CAD build for the part. Positions are in the model's coordinates, mm. A direction names the side the tool comes from. Coordinates: 2 decimals unless noted, no trailing zeros. Write each loop counter-clockwise with the first axis right and the second up, starting at its lowest first coordinate (ties: lowest second). Pieces come first, ordered by that corner, then holes. Notation, with made-up numbers: (-34, -1.5) - (2, -1.5) arc R14 ccw to (2, 16.5) - close; hole circle Ø1 at (-18, 0). An arc over 180 degrees is marked (long way). Answer in a Markdown table with one row per item. Add a question column.
Q1. Two-plate mould, pull along Z, no slides. Class faces 6 (the cylindrical face through (26.36, 3.9, -5.13)), 7 (the cylindrical face through (-12.15, 49.02, -13.91)), 8 (the cylindrical face through (17.483, 49.021, -0.26)): +Z half, -Z half, draft (parallel to the pull), parting line (faces both ways), or undercut.
Q2. Pin check, flat tips, straight feed: pin 1 (5.5 mm diameter, centred on y = 29.5, z = -3.5, fed in from +X); pin 2 (1.5 mm diameter, centred on y = 7.5, z = -11.5, fed in from -X); pin 3 (5.5 mm diameter, centred on x = -34.5, z = -9.5, fed in from +Y). Stop position of each tip, or through.
Q3. Drill centre lines: line 1 along X through (y, z) = (48.9, 0); line 2 along X through (y, z) = (44.5, -6.5); line 3 along X through (y, z) = (1, -5). Where is each one in solid material? Low to high. Write a range as from..to.
Q4. 3-axis set-ups, long thin cutter, end or side, ignore diameter. For faces 1 (the cylindrical face through (38, 2, -5)), 2 (the flat face through (36, 3, -5)), 3 (the flat face through (22.5, 25, -5)), 4 (the cylindrical face through (12.11, 49.02, -13.88)), 5 (the flat face through (-36, 3, -5)): which of +Z, -Z, +X, -X, +Y, -Y reach the whole face in a straight line?
Q5. Band-saw the part on B-B (x = 40). List the corners of the cut face in (y, z).
Q6. Band-saw the part on C-C (z = -0.5). List the corners of the cut face in (x, y), and give its area (3 significant figures).
Q7. Band-saw the part on A-A (y = 33.5). List the corners of the cut face in (x, z).
Q8. Band-saw the part on D-D (z = -9.25). List the corners of the cut face in (x, y), and give its area (3 significant figures).
```python
from build123d import *

# Parameters (mm, degrees)
EXTRUDE_THIN1_DEPTH = 4.5
SKETCH2_R           = 2
CUT_EXTRUDE1_DEPTH  = 70.474815581
BOSS_EXTRUDE1_DEPTH = 10
SKETCH4_R           = 11.5
CUT_EXTRUDE2_DEPTH  = 71.829019476
FILLET1_R           = 3
FILLET2_R           = 3
SKETCH5_R           = 2
CUT_EXTRUDE3_DEPTH  = 69.722267134


with BuildPart() as part:
    # Sketch1 → Extrude-Thin1 (new, symmetric)
    with BuildSketch(Plane.XY):
        Polygon((-47.5, 0), (-22.5, 0), (-22.5, 47.5), (0, 47.5), (0, 50.5), (-25.5, 50.5), (-25.5, 3), (-47.5, 3), align=None)
    extrude_thin1 = extrude(amount=EXTRUDE_THIN1_DEPTH, both=True)

    # Mirror1: Extrude-Thin1 across plane
    add(extrude_thin1.mirror(Plane(origin=(0, 50.5, 4.5), x_dir=(0, 0, 1), z_dir=(1, 0, 0))))

    # Sketch2 → Cut-Extrude1 (cut, through all)
    with BuildSketch(Plane(origin=(0, 50.5, 0), x_dir=(1, 0, 0), z_dir=(0, 1, 0))):
        with Locations(Location((-15.5, 0, 0), (0, 0, 270))):
            Circle(SKETCH2_R)
        with Locations(Location((15.5, 0, 0), (0, 0, 270))):
            Circle(SKETCH2_R)
    extrude(amount=-CUT_EXTRUDE1_DEPTH, mode=Mode.SUBTRACT)

    # Sketch3 → Boss-Extrude1 (add)
    with BuildSketch(Plane(origin=(0, 0, -4.5), x_dir=(-1, 0, 0), z_dir=(0, 0, -1))):
        Polygon((-22.5, 47.5), (22.5, 47.5), (22.5, 0), (47.5, 0), (47.5, 3), (25.5, 3), (25.5, 50.5), (-25.5, 50.5), (-25.5, 3), (-47.5, 3), (-47.5, 0), (-22.5, 0), align=None)
    extrude(amount=BOSS_EXTRUDE1_DEPTH)

    # Sketch4 → Cut-Extrude2 (cut, through all)
    with BuildSketch(Plane(origin=(0, 50.5, 0), x_dir=(1, 0, 0), z_dir=(0, 1, 0))):
        with Locations((0, 15.5)):
            Circle(SKETCH4_R)
    extrude(amount=-CUT_EXTRUDE2_DEPTH, mode=Mode.SUBTRACT)

    # Fillet1
    fillet1_edges = [part.edges().sort_by_distance(p)[0] for p in [
        (-11.456439237, 49, -14.5),
        (11.456439237, 49, -14.5),
    ]]
    fillet(fillet1_edges, radius=FILLET1_R)

    # Fillet2
    fillet2_edges = [part.edges().sort_by_distance(p)[0] for p in [
        (-22.5, 0, -5),
        (-25.5, 3, -5),
        (22.5, 0, -5),
        (25.5, 3, -5),
    ]]
    fillet(fillet2_edges, radius=FILLET2_R)

    # Sketch5 → Cut-Extrude3 (cut, through all)
    with BuildSketch(Plane(origin=(0, 3, 0), x_dir=(1, 0, 0), z_dir=(0, 1, 0))):
        with Locations(Location((-40, 5, 0), (0, 0, 270))):
            Circle(SKETCH5_R)
        with Locations(Location((40, 5, 0), (0, 0, 270))):
            Circle(SKETCH5_R)
    extrude(amount=-CUT_EXTRUDE3_DEPTH, mode=Mode.SUBTRACT)


solid = part.part
```
Checked values:
| question | item | result |
|---|---|---|
| 1 | face 6 | draft |
| 1 | face 7 | -Z half |
| 1 | face 8 | undercut |
| 2 | pin 1 | stops at x = 25.5 |
| 2 | pin 2 | stops at x = -25.5 |
| 2 | pin 3 | stops at y = 3 |
| 3 | line 1 | x = -25.5..-17.5, -13.5..13.5, 17.5..25.5 |
| 3 | line 2 | x = -25.5..-22.5, 22.5..25.5 |
| 3 | line 3 | x = -47.5..-42, -38..-23.26, 23.26..38, 42..47.5 |
| 4 | face 1 | +Y, -Y |
| 4 | face 2 | +Z, -Z, +X, +Y |
| 4 | face 3 | +Z, -Z, -Y |
| 4 | face 4 | -Z, +Y, -Y |
| 4 | face 5 | +Z, -Z, -X, +Y |
| 5 | outline | (0, -14.5) - (3, -14.5) - (3, -7) - (0, -7) - close; (0, -3) - (3, -3) - (3, 4.5) - (0, 4.5) - close |
| 6 | outline | (-47.5, 0) - (-25.5, 0) arc R3 ccw to (-22.5, 3) - (-22.5, 47.5) - (-17.44, 47.5) - (-17.44, 50.5) - (-25.5, 50.5) - (-25.5, 6) arc R3 cw to (-28.5, 3) - (-47.5, 3) - close; (-13.56, 47.5) - (13.56, 47.5) - (13.56, 50.5) - (-13.56, 50.5) - close; (17.44, 47.5) - (22.5, 47.5) - (22.5, 3) arc R3 ccw to (25.5, 0) - (47.5, 0) - (47.5, 3) - (28.5, 3) arc R3 cw to (25.5, 6) - (25.5, 50.5) - (17.44, 50.5) - close |
| 6 | area | 547 mm² |
| 7 | outline | (-25.5, -14.5) - (-22.5, -14.5) - (-22.5, 4.5) - (-25.5, 4.5) - close; (22.5, -14.5) - (25.5, -14.5) - (25.5, 4.5) - (22.5, 4.5) - close |
| 8 | outline | (-47.5, 0) - (-25.5, 0) arc R3 ccw to (-22.5, 3) - (-22.5, 47.5) - (-9.65, 47.5) - (-9.65, 50.5) - (-25.5, 50.5) - (-25.5, 6) arc R3 cw to (-28.5, 3) - (-47.5, 3) - close; (9.65, 47.5) - (22.5, 47.5) - (22.5, 3) arc R3 ccw to (25.5, 0) - (47.5, 0) - (47.5, 3) - (28.5, 3) arc R3 cw to (25.5, 6) - (25.5, 50.5) - (9.65, 50.5) - close |
| 8 | area | 512 mm² |
